Model file for the job. Use its own axes, mm. Face numbers are marked on the shaded views. A direction names the side the tool comes from. Round coordinates to 2 decimals unless told otherwise and drop trailing zeros. Order: outer loops, then holes, each group sorted by start corner. A loop starts at its lowest first (then second) coordinate and runs counter-clockwise, first axis right, second up. Notation, with made-up numbers: (22, 81) -> (62, 81) arc R31 cw to (62, 111) -> close; hole circle Ø9 at (27, 22). An arc over 180 degrees is marked (long way). Answer as CSV lines item,"result".
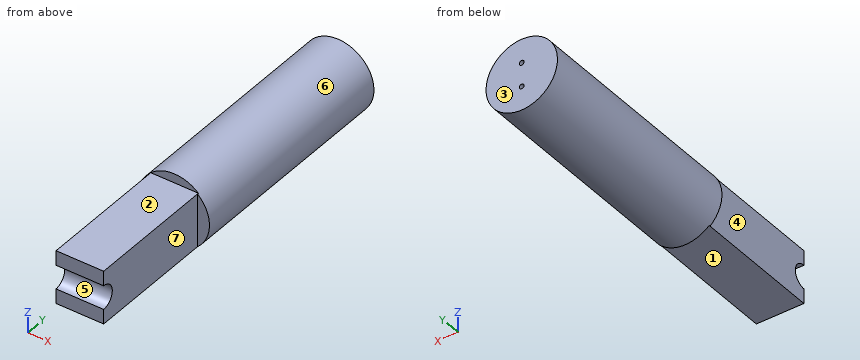
```python
from build123d import *

# Parameters (mm, degrees)
SKETCH2_R           = 15
BOSS_EXTRUDE1_DEPTH = 150
CUT_EXTRUDE1_START  = 10
SKETCH3_W           = 30
SKETCH3_H           = 108.98871412
CUT_EXTRUDE1_DEPTH  = 100
CUT_EXTRUDE2_START  = -10
SKETCH3_2_W         = 30
SKETCH3_2_H         = 108.98871412
CUT_EXTRUDE2_DEPTH  = 100
CUT_EXTRUDE4_DEPTH  = 55
SKETCH4_R           = 5
CUT_EXTRUDE5_DEPTH  = 153.807067899
SKETCH6_R           = 1
CUT_EXTRUDE6_DEPTH  = 8


with BuildPart() as part:
    # Sketch2 → Boss-Extrude1 (new body)
    with BuildSketch(Plane(origin=(0, 0, 0), x_dir=(1, 0, 0), z_dir=(0, 1, 0))):
        with Locations(Location((0, 0, 0), (0, 0, 270))):
            Circle(SKETCH2_R)
    extrude(amount=BOSS_EXTRUDE1_DEPTH)

    # Sketch3 → Cut-Extrude1 (cut)
    with BuildSketch(Plane(origin=(0, 0, 0), x_dir=(0, 0, -1), z_dir=(1, 0, 0)).offset(CUT_EXTRUDE1_START)):
        Rectangle(SKETCH3_W, SKETCH3_H)
    extrude(amount=CUT_EXTRUDE1_DEPTH, mode=Mode.SUBTRACT)

    # Sketch3_2 → Cut-Extrude2 (cut)
    with BuildSketch(Plane(origin=(0, 0, 0), x_dir=(0, 0, -1), z_dir=(1, 0, 0)).offset(CUT_EXTRUDE2_START)):
        Rectangle(SKETCH3_2_W, SKETCH3_2_H)
    extrude(amount=-CUT_EXTRUDE2_DEPTH, mode=Mode.SUBTRACT)

    # Sketch5 → Cut-Extrude4 (cut)
    with BuildSketch(Plane.XZ):
        with BuildLine():
            Line((-10, 11.180339887), (10, 11.180339887))
            ThreePointArc((10, 11.180339887), (0, 15), (-10, 11.180339887))
        make_face()
        with BuildLine():
            Line((-10, -11.180339887), (10, -11.180339887))
            ThreePointArc((10, -11.180339887), (0, -15), (-10, -11.180339887))
        make_face()
    extrude(amount=-CUT_EXTRUDE4_DEPTH, mode=Mode.SUBTRACT)

    # Sketch4 → Cut-Extrude5 (cut, through all)
    with BuildSketch(Plane(origin=(10, 0, 0), x_dir=(0, 0, -1), z_dir=(1, 0, 0))):
        with Locations((0.000339887, 0)):
            Circle(SKETCH4_R)
    extrude(amount=-CUT_EXTRUDE5_DEPTH, mode=Mode.SUBTRACT)

    # Sketch6 → Cut-Extrude6 (cut)
    with BuildSketch(Plane(origin=(0, 150, 0), x_dir=(1, 0, 0), z_dir=(0, 1, 0))):
        with Locations(Location((0, 5, 0), (0, 0, 270))):
            Circle(SKETCH6_R)
        with Locations(Location((0, -5, 0), (0, 0, 270))):
            Circle(SKETCH6_R)
    extrude(amount=-CUT_EXTRUDE6_DEPTH, mode=Mode.SUBTRACT)


solid = part.part
```
Q1. Saw through at C-C (y = 29). Write the cut outline in (x, z).
Checks:
outline,"(-10, -11.18) -> (10, -11.18) -> (10, 11.18) -> (-10, 11.18) -> close"
Q2. Flat gauge pins, fed straight in: pin 1 (1 mm diameter, centred on y = 113.5, z = -11, fed in from -X); pin 2 (1.5 mm diameter, centred on x = -13.5, z = 0.5, fed in from -Y); pin 3 (11 mm diameter, centred on y = 34.5, z = 3, fed in from -X). Where does each tip first touch, or does it go through?
Checks:
pin 1,"x = -10.71"
pin 2,"y = 54.49"
pin 3,"x = -10"
Q3. Tool access for the marked faces 1, 2, 3 and 4: list every direction of +Z, -Z, +X, -X, +Y, -Y with a clear straight run to the whole face (end or side of a thin tool).
Checks:
face 1,"-Z, +X, -X, -Y"
face 2,"+Z, +X, -X, -Y"
face 3,"+Z, -Z, +X, -X, +Y"
face 4,"+Z, -Z, -X, -Y"
Q4. Saw through at D-D (y = 125.5). Write the cut outline in (x, z), plus the area to 3 significant figures.
Checks:
outline,"circle Ø30 at (0, 0)"
area,"707 mm²"
Q5. Wall check: L1, parallel to Y at x = 12.25, z = 4.5; L2, parallel to Z at x = -2, y = 30; L3, parallel to X at y = 11, z = 1. Give the ranges that are in metal, low to high. Write a range as [from, to].
Checks:
L1,"[54.49, 150]"
L2,"[-11.18, 11.18]"
L3,"[-10, 10]"
Q6. Mould opens along Z. For the marked faces 5, 6 and 7 say: +Z half, -Z half, draft (parallel to the pull), parting line (faces both ways), or undercut.
Checks:
face 5,"undercut"
face 6,"parting line"
face 7,"draft"
Q7. Saw through at B-B (x = 5.5). Write the cut outline in (y, z), plus the area to 3 significant figures.
Checks:
outline,"(0, -11.18) -> (55, -11.18) -> (55, -13.96) -> (150, -13.96) -> (150, 13.96) -> (55, 13.96) -> (55, 11.18) -> (0, 11.18) -> (0, 5) arc R5 cw to (0, -5) -> close"
area,"3,840 mm²"
Q8. Saw through at A-A (z = 0). Write the cut outline in (x, y).
Checks:
outline,"(-15, 54.49) -> (-10, 54.49) -> (-10, 5) -> (10, 5) -> (10, 54.49) -> (15, 54.49) -> (15, 150) -> (-15, 150) -> close"
